```python
from build123d import *

# Parameters (mm, degrees)
SKETCH1_W           = 2100
SKETCH1_H           = 1150
SKETCH1_W_2         = 1980
SKETCH1_H_2         = 1000
BOSS_EXTRUDE1_DEPTH = 30
SKETCH2_R           = 6.35
CUT_EXTRUDE1_DEPTH  = 1198.507828784


with BuildPart() as part:
    # Sketch1 → Boss-Extrude1 (new body)
    with BuildSketch(Plane(origin=(0, 0, 0), x_dir=(1, 0, 0), z_dir=(0, 1, 0))):
        Rectangle(SKETCH1_W, SKETCH1_H)
        Rectangle(SKETCH1_W_2, SKETCH1_H_2, mode=Mode.SUBTRACT)
    extrude(amount=-BOSS_EXTRUDE1_DEPTH)

    # Sketch2 → Cut-Extrude1 (cut, through all)
    with BuildSketch(Plane(origin=(0, 0, 0), x_dir=(1, 0, 0), z_dir=(0, 1, 0))):
        with Locations(Location((-1020, 545, 0), (0, 0, 270))):
            Circle(SKETCH2_R)
        with Locations(Location((-1020, -545, 0), (0, 0, 270))):
            Circle(SKETCH2_R)
        with Locations(Location((1020, 545, 0), (0, 0, 270))):
            Circle(SKETCH2_R)
        with Locations(Location((1020, -545, 0), (0, 0, 270))):
            Circle(SKETCH2_R)
    extrude(amount=-CUT_EXTRUDE1_DEPTH, mode=Mode.SUBTRACT)


solid = part.part
```
Check sheet for the modelled part. Datum: model origin and axes. Units: mm. Coordinates: 2 decimals unless noted, no trailing zeros. Loops run counter-clockwise (first coordinate to the right, second up) from the corner with the lowest first, then second, coordinate; pieces in that order, holes last. Notation, with made-up numbers: M -37.5,71.25 L -31.5,71.25 A5 cw -31.5,80.25 Z; hole C 34,-29.75 d9. An arc over 180 degrees is marked long. Answer as a JSON object with one key per item and string values.
1. Sectioned sample at B-B on y = -17. Record the cut outline in (x, z), and give its area (3 significant figures).
Outcome:
{"outline": "M -1050,-575 L 1050,-575 L 1050,575 L -1050,575 Z; hole C -1020,-545 d12.7; hole C -1020,545 d12.7; hole M -990,-500 L 990,-500 L 990,500 L -990,500 Z; hole C 1020,-545 d12.7; hole C 1020,545 d12.7", "area": "434,000 mm²"}
2. Sectioned sample at C-C on x = 300.5. Record the cut outline in (y, z).
Outcome:
{"outline": "M -30,-575 L 0,-575 L 0,-500 L -30,-500 Z; M -30,500 L 0,500 L 0,575 L -30,575 Z"}
3. Scan lines: L1, parallel to X at y = -19.25, z = 545; L2, parallel to Z at x = -1020, y = -6.25; L3, parallel to Z at x = -45.5, y = -5.5. Record each from-to range of solid material in increasing order. Write a range as from..to.
Outcome:
{"L1": "-1050..-1026.35, -1013.65..1013.65, 1026.35..1050", "L2": "-575..-551.35, -538.65..538.65, 551.35..575", "L3": "-575..-500, 500..575"}
4. Depth check by flat-ended pin: P1, Ø7.5, axis at x = -1020, z = 545, coming from the -Y side. Enter the tip coordinate at first touch or a pass-through.
Outcome:
{"P1": "through"}
5. Sectioned sample at A-A on z = 468. Record the cut outline in (x, y), and give its area (3 significant figures).
Outcome:
{"outline": "M -1050,-30 L -990,-30 L -990,0 L -1050,0 Z; M 990,-30 L 1050,-30 L 1050,0 L 990,0 Z", "area": "3,600 mm²"}
